Verification items for the finished model (mm, model axes). Face numbers are marked on the shaded views. A direction names the side the tool comes from. Give positions to 0.01 mm unless a question says otherwise; leave off trailing zeros. Order: outer loops, then holes, each group sorted by start corner. A loop starts at its lowest first (then second) coordinate and runs counter-clockwise, first axis right, second up. Notation, with made-up numbers: (65, 85) -> (120, 85) arc R32 ccw to (120, 118) -> close; hole circle Ø7 at (48.25, 65). An arc over 180 degrees is marked (long way). Write each question's results on one line, items separated by ' | '. Start each with the question number.
1. Cross-section at B-B, the plane y = -39.5. Enter the section's corners in (x, z), then the cut area to 3 significant figures.
2. Depth check by flat-ended pin: pin 1 Ø4 at (x, y) = (-64, -120) entering from +Z; pin 2 Ø10 at (x, z) = (18, -124.5) entering from +Y; pin 3 Ø2 at (x, y) = (23.5, -29) entering from -Z. Enter the tip coordinate at first touch or a pass-through.
3. Cross-section at C-C, the plane z = -99. Enter the section's corners in (x, y).
4. Material ranges on L1, parallel to Y at x = 64, z = 26; L2, parallel to X at y = 180, z = 23; L3, parallel to Z at x = 45.5, y = -109, recorded low to high. Write a range as from..to.
5. Cross-section at D-D, the plane y = 159.5. Enter the section's corners in (x, z).
6. Cross-section at A-A, the plane x = 40.5. Enter the section's corners in (y, z).
7. Set-up check for the marked faces 1, 2 and 3: record each of +Z, -Z, +X, -X, +Y, -Y from which the full face is reachable in a straight line by a thin tool's end or side.
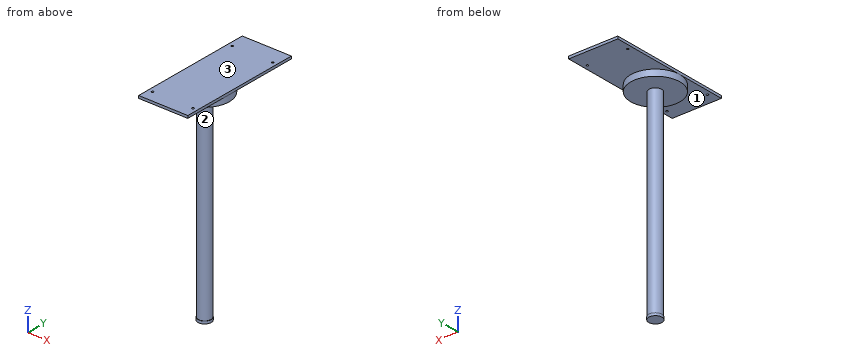
Autodesk Inventor part; units mm, degrees
ref_plane "YZ Plane" through (0, 0, 0) normal (1, 0, 0) x (0, 1, 0)
ref_plane "XZ Plane" through (0, 0, 0) normal (0, 1, 0) x (-1, 0, 0)
ref_plane "XY Plane" through (0, 0, 0) normal (0, 0, 1) x (1, 0, 0)
sketch "Sketch1" plane through (0, 0, 0) normal (0, 0, 1) x (1, 0, 0)
  circle A0 centre (0, 0) radius 78
extrude "Connector" add sketch "Sketch1" along normal blind 20
sketch "Sketch2" plane through (0, 0, 0) normal (0, 0, -1) x (-1, 0, 0)
  circle A0 centre (0, 0) radius 20
extrude "RotAxis" add sketch "Sketch2" along normal blind 624
sketch "Sketch3" plane through (0, 0, 20) normal (0, 0, 1) x (1, 0, 0)
  line L0 (78, 234) -> (-78, 234)
  line L1 (-78, 234) -> (-78, -156)
  line L2 (-78, -156) -> (78, -156)
  line L3 (78, -156) -> (78, 234)
  point P0 (0, 0)
extrude "TelescopeMount" add sketch "Sketch3" along normal blind 8
sketch "Sketch4" plane through (0, 0, -624) normal (0, 0, -1) x (-1, 0, 0)
  circle A0 centre (0, 0) radius 21
extrude "Cap" add sketch "Sketch4" along normal blind 8
sketch "Sketch5" plane through (0, 0, 28) normal (0, 0, 1) x (1, 0, 0)
  line L0 (-78, 234) -> (-78, -156)
  line L1 (78, -156) -> (78, 234)
  point P0 (0, 0)
  point P1 (64, -120)
  point P2 (-64, -120)
  point P3 (-64, 180)
  point P4 (64, 180)
hole "Hole1" at (64, -120, 28) at (-64, -120, 28) at (-64, 180, 28) at (64, 180, 28) direction (0, 0, -1) diameter 6.647 end through all
properties part number "DecAxis"
Results below:
1) outline: (-78, 20) -> (-67.26, 20) -> (-67.26, 0) -> (67.26, 0) -> (67.26, 20) -> (78, 20) -> (78, 28) -> (-78, 28) -> close | area: 3,940 mm²
2) pin 1: passes through | pin 2: stops at y = 15.2 | pin 3: stops at z = 0
3) outline: circle Ø40 at (0, 0)
4) L1: y = -156..-123.32, -116.68..176.68, 183.32..234 | L2: x = -78..-67.32, -60.68..60.68, 67.32..78 | L3: z = 20..28
5) outline: (-78, 20) -> (78, 20) -> (78, 28) -> (-78, 28) -> close
6) outline: (-156, 20) -> (-66.66, 20) -> (-66.66, 0) -> (66.66, 0) -> (66.66, 20) -> (234, 20) -> (234, 28) -> (-156, 28) -> close
7) face 1: -Z, -Y | face 2: none | face 3: +Z, +X, -X, +Y, -Y
